from build123d import *

# Parameters (mm, degrees)
SKETCH1_W            = 114.4
SKETCH1_H            = 94.4
BOSS_EXTRUDE1_DEPTH  = 10
SHELL2_T             = -2
FILLET3_R            = 5
FILLET4_R            = 5
SKETCH5_R            = 4
BOSS_EXTRUDE12_DEPTH = 8
FILLET5_R            = 5
FILLET6_R            = 5
FILLET7_R            = 5
FILLET8_R            = 5
FILLET9_R            = 5
FILLET10_R           = 5
FILLET11_DEPTH       = 9
FILLET12_DEPTH       = 9
SKETCH6_R            = 1.6
CUT_EXTRUDE1_DEPTH   = 10
SKETCH7_R            = 4
BOSS_EXTRUDE13_DEPTH = 10
SKETCH8_R            = 1.5
CUT_EXTRUDE2_DEPTH   = 8
SKETCH9_R            = 2.5
CUT_EXTRUDE3_DEPTH   = 2


with BuildPart() as part:
    # Sketch1 → Boss-Extrude1 (new body)
    with BuildSketch(Plane(origin=(0, 0, 0), x_dir=(1, 0, 0), z_dir=(0, 1, 0))):
        with Locations((57.2, 47.2)):
            Rectangle(SKETCH1_W, SKETCH1_H)
    extrude(amount=BOSS_EXTRUDE1_DEPTH)

    # Shell2
    shell2_openings = [part.faces().sort_by_distance(p)[0] for p in [
        (57.2, 0, -47.2),
    ]]
    offset(amount=SHELL2_T, openings=shell2_openings, kind=Kind.INTERSECTION)

    # Fillet3
    fillet3_edges = [part.edges().sort_by_distance(p)[0] for p in [
        (0, 5, -94.4),
        (114.4, 5, -94.4),
        (114.4, 5, 0),
        (0, 5, 0),
    ]]
    fillet(fillet3_edges, radius=FILLET3_R)

    # Fillet4
    fillet4_edges = [part.edges().sort_by_distance(p)[0] for p in [
        (2, 4, -92.4),
        (2, 4, -2),
        (112.4, 4, -2),
        (112.4, 4, -92.4),
    ]]
    fillet(fillet4_edges, radius=FILLET4_R)

    # Sketch5 → Boss-Extrude12 (add)
    with BuildSketch(Plane(origin=(0, 8, 0), x_dir=(-1, 0, 0), z_dir=(0, -1, 0))):
        with Locations((-108.4, 6)):
            Circle(SKETCH5_R)
        with Locations((-108.4, 88.4)):
            Circle(SKETCH5_R)
        with Locations((-6, 88.4)):
            Circle(SKETCH5_R)
        with Locations((-6, 6)):
            Circle(SKETCH5_R)
    extrude(amount=BOSS_EXTRUDE12_DEPTH)

    # Fillet5
    # the kernel refuses this fillet: 5 mm, written as the material it adds along each edge
    with BuildSketch(Plane(origin=(112.372048604, 0, -6.472048604), x_dir=(-0.783459029597643, 0, -0.6214434398574978), z_dir=(0, 1, 0))) as fillet5_piece_1_section:
        with BuildLine():
            CenterArc((9.160403969, -3.547792862), FILLET5_R, 134.800989095, 83.620629792)
            Line((5.243108821, -6.655010061), (4.851379306, -6.965731781))
            ThreePointArc((4.851379306, -6.965731781), (-0.085536357, -0.74172022), (-0.422348831, -0.26762187))
            Line((-0.422348831, -0.26762187), (0.35232323, 0.354779286))
            ThreePointArc((0.35232323, 0.354779286), (2.818585837, -0.661765711), (5.284848444, 0.354779286))
            Line((5.284848444, 0.354779286), (5.637171673, 0))
        make_face()
    fillet5_piece_1 = extrude(amount=29.180673535, mode=Mode.PRIVATE)
    fillet5_piece_1 = split(fillet5_piece_1, bisect_by=Plane(origin=(112.372048604, 10, -6.472048604), z_dir=(0, -1, 0)), keep=Keep.TOP, mode=Mode.PRIVATE)
    add(fillet5_piece_1)

    # Fillet6
    # the kernel refuses this fillet: 5 mm, written as the material it adds along each edge
    with BuildSketch(Plane(origin=(107.927951396, 0, -2.027951396), x_dir=(-0.6214434398574917, 0, -0.7834590295976479), z_dir=(0, 1, 0))) as fillet6_piece_1_section:
        with BuildLine():
            CenterArc((9.160403969, 3.547792862), FILLET6_R, 141.578381114, 83.620629792)
            Line((5.243108821, 6.655010061), (4.851379306, 6.965731781))
            ThreePointArc((4.851379306, 6.965731781), (-0.085536357, 0.74172022), (-0.422348831, 0.26762187))
            Line((-0.422348831, 0.26762187), (0.35232323, -0.354779286))
            ThreePointArc((0.35232323, -0.354779286), (2.818585837, 0.661765711), (5.284848444, -0.354779286))
            Line((5.284848444, -0.354779286), (5.637171673, 0))
        make_face()
    fillet6_piece_1 = extrude(amount=29.180673535, mode=Mode.PRIVATE)
    fillet6_piece_1 = split(fillet6_piece_1, bisect_by=Plane(origin=(107.927951396, 10, -2.027951396), z_dir=(0, -1, 0)), keep=Keep.TOP, mode=Mode.PRIVATE)
    add(fillet6_piece_1)

    # Fillet7
    # the kernel refuses this fillet: 5 mm, written as the material it adds along each edge
    with BuildSketch(Plane(origin=(112.372048604, 0, -87.927951396), x_dir=(-0.783459029597643, 0, 0.6214434398574978), z_dir=(0, 1, 0))) as fillet7_piece_1_section:
        with BuildLine():
            CenterArc((9.160403969, 3.547792862), FILLET7_R, 141.578381114, 83.620629792)
            Line((5.243108821, 6.655010061), (4.851379306, 6.965731781))
            ThreePointArc((4.851379306, 6.965731781), (-0.085536357, 0.74172022), (-0.422348831, 0.26762187))
            Line((-0.422348831, 0.26762187), (0.35232323, -0.354779286))
            ThreePointArc((0.35232323, -0.354779286), (2.818585837, 0.661765711), (5.284848444, -0.354779286))
            Line((5.284848444, -0.354779286), (5.637171673, 0))
        make_face()
    fillet7_piece_1 = extrude(amount=29.180673535, mode=Mode.PRIVATE)
    fillet7_piece_1 = split(fillet7_piece_1, bisect_by=Plane(origin=(112.372048604, 10, -87.927951396), z_dir=(0, -1, 0)), keep=Keep.TOP, mode=Mode.PRIVATE)
    add(fillet7_piece_1)

    # Fillet8
    # the kernel refuses this fillet: 5 mm, written as the material it adds along each edge
    with BuildSketch(Plane(origin=(107.927951396, 0, -92.372048604), x_dir=(-0.6214434398574917, 0, 0.7834590295976479), z_dir=(0, 1, 0))) as fillet8_piece_1_section:
        with BuildLine():
            CenterArc((9.160403969, -3.547792862), FILLET8_R, 134.800989095, 83.620629792)
            Line((5.243108821, -6.655010061), (4.851379306, -6.965731781))
            ThreePointArc((4.851379306, -6.965731781), (-0.085536357, -0.74172022), (-0.422348831, -0.26762187))
            Line((-0.422348831, -0.26762187), (0.35232323, 0.354779286))
            ThreePointArc((0.35232323, 0.354779286), (2.818585837, -0.661765711), (5.284848444, 0.354779286))
            Line((5.284848444, 0.354779286), (5.637171673, 0))
        make_face()
    fillet8_piece_1 = extrude(amount=29.180673535, mode=Mode.PRIVATE)
    fillet8_piece_1 = split(fillet8_piece_1, bisect_by=Plane(origin=(107.927951396, 10, -92.372048604), z_dir=(0, -1, 0)), keep=Keep.TOP, mode=Mode.PRIVATE)
    add(fillet8_piece_1)

    # Fillet9
    # the kernel refuses this fillet: 5 mm, written as the material it adds along each edge
    with BuildSketch(Plane(origin=(6.472048604, 29.180673535, -2.027951396), x_dir=(0.9999945577477605, 0, 0.003299162751511756), z_dir=(0, -1, 0))) as fillet9_piece_1_section:
        with BuildLine():
            CenterArc((8.4557736, -4.999972789), FILLET9_R, 89.810971555, 83.620629792)
            Line((3.488593561, -4.428026585), (2.991875557, -4.370831965))
            ThreePointArc((2.991875557, -4.370831965), (2.264117061, -1.804476076), (-0.060643809, -0.496308703))
            Line((-0.060643809, -0.496308703), (-0.051154492, 0.497376334))
            ThreePointArc((-0.051154492, 0.497376334), (0.52969032, 0.526206725), (8.473918995, 0.499997279))
            Line((8.473918995, 0.499997279), (8.472269414, 0))
        make_face()
    fillet9_piece_1 = extrude(amount=29.180673535, mode=Mode.PRIVATE)
    fillet9_piece_1 = split(fillet9_piece_1, bisect_by=Plane(origin=(6.472048604, 10, -2.027951396), z_dir=(0, -1, 0)), keep=Keep.TOP, mode=Mode.PRIVATE)
    add(fillet9_piece_1)

    # Fillet10
    # the kernel refuses this fillet: 5 mm, written as the material it adds along each edge
    with BuildSketch(Plane(origin=(2.027951396, 29.180673535, -6.472048604), x_dir=(0.783459029597646, 0, -0.6214434398574942), z_dir=(0, -1, 0))) as fillet10_piece_1_section:
        with BuildLine():
            CenterArc((9.160403969, -3.547792862), FILLET10_R, 134.800989095, 83.620629792)
            Line((5.243108821, -6.655010061), (4.851379306, -6.965731781))
            ThreePointArc((4.851379306, -6.965731781), (-0.085536357, -0.74172022), (-0.422348831, -0.26762187))
            Line((-0.422348831, -0.26762187), (0.35232323, 0.354779286))
            ThreePointArc((0.35232323, 0.354779286), (2.818585837, -0.661765711), (5.284848444, 0.354779286))
            Line((5.284848444, 0.354779286), (5.637171673, 0))
        make_face()
    fillet10_piece_1 = extrude(amount=29.180673535, mode=Mode.PRIVATE)
    fillet10_piece_1 = split(fillet10_piece_1, bisect_by=Plane(origin=(2.027951396, 10, -6.472048604), z_dir=(0, -1, 0)), keep=Keep.TOP, mode=Mode.PRIVATE)
    add(fillet10_piece_1)

    # Fillet11: read off the stored shape, not the designer's step
    # Fillet11 outline → Fillet11 (add)
    with BuildSketch(Plane(origin=(0, 0, 0), x_dir=(1, 0, 0), z_dir=(0, 1, 0))):
        with BuildLine():
            ThreePointArc((2, 79.45572809), (3.273220038, 82.789061423), (6.444444444, 84.42476804))
            ThreePointArc((6.444444444, 84.42476804), (3.51422624, 85.266163882), (2.027951396, 87.927951396))
            ThreePointArc((2.027951396, 87.927951396), (2.006992739, 87.664345398), (2, 87.4))
            Line((2, 87.4), (2, 79.45572809))
        make_face()
    extrude(amount=FILLET11_DEPTH)

    # Fillet12: read off the stored shape, not the designer's step
    # Fillet12 outline → Fillet12 (add)
    with BuildSketch(Plane(origin=(0, 0, 0), x_dir=(1, 0, 0), z_dir=(0, 1, 0))):
        with BuildLine():
            ThreePointArc((9.97523196, 87.955555556), (11.610938577, 91.126779962), (14.94427191, 92.4))
            Line((14.94427191, 92.4), (7, 92.4))
            ThreePointArc((7, 92.4), (6.735654602, 92.393007261), (6.472048604, 92.372048604))
            ThreePointArc((6.472048604, 92.372048604), (9.133836118, 90.88577376), (9.97523196, 87.955555556))
        make_face()
    extrude(amount=FILLET12_DEPTH)

    # Sketch6 → Cut-Extrude1 (cut)
    with BuildSketch(Plane(origin=(0, 0, 0), x_dir=(-1, 0, 0), z_dir=(0, -1, 0))):
        with Locations(Location((-6, 6, 0), (0, 0, 90))):
            Circle(SKETCH6_R)
        with Locations(Location((-108.4, 88.4, 0), (0, 0, 90))):
            Circle(SKETCH6_R)
        with Locations(Location((-108.4, 6, 0), (0, 0, 90))):
            Circle(SKETCH6_R)
        with Locations(Location((-6, 88.4, 0), (0, 0, 90))):
            Circle(SKETCH6_R)
    extrude(amount=-CUT_EXTRUDE1_DEPTH, mode=Mode.SUBTRACT)

    # Sketch7 → Boss-Extrude13 (add)
    with BuildSketch(Plane(origin=(0, 8, 0), x_dir=(-1, 0, 0), z_dir=(0, -1, 0))):
        with Locations(Location((-96.5, 19.1, 0), (0, 0, 90))):
            Circle(SKETCH7_R)
        with Locations(Location((-17, 19.1, 0), (0, 0, 90))):
            Circle(SKETCH7_R)
        with Locations(Location((-96.5, 77.4, 0), (0, 0, 90))):
            Circle(SKETCH7_R)
        with Locations(Location((-17, 77.4, 0), (0, 0, 90))):
            Circle(SKETCH7_R)
    extrude(amount=BOSS_EXTRUDE13_DEPTH)

    # Sketch8 → Cut-Extrude2 (cut)
    with BuildSketch(Plane(origin=(0, -2, 0), x_dir=(-1, 0, 0), z_dir=(0, -1, 0))):
        with Locations(Location((-17, 19.1, 0), (0, 0, 90))):
            Circle(SKETCH8_R)
        with Locations(Location((-96.5, 19.1, 0), (0, 0, 90))):
            Circle(SKETCH8_R)
        with Locations(Location((-96.5, 77.4, 0), (0, 0, 90))):
            Circle(SKETCH8_R)
        with Locations(Location((-17, 77.4, 0), (0, 0, 90))):
            Circle(SKETCH8_R)
    extrude(amount=-CUT_EXTRUDE2_DEPTH, mode=Mode.SUBTRACT)

    # Sketch9 → Cut-Extrude3 (cut)
    with BuildSketch(Plane(origin=(0, 10, 0), x_dir=(1, 0, 0), z_dir=(0, 1, 0))):
        with Locations(Location((6, 88.4, 0), (0, 0, 270))):
            Circle(SKETCH9_R)
        with Locations(Location((6, 6, 0), (0, 0, 270))):
            Circle(SKETCH9_R)
        with Locations(Location((108.4, 6, 0), (0, 0, 270))):
            Circle(SKETCH9_R)
        with Locations(Location((108.4, 88.4, 0), (0, 0, 270))):
            Circle(SKETCH9_R)
    extrude(amount=-CUT_EXTRUDE3_DEPTH, mode=Mode.SUBTRACT)


solid = part.part
Geometry check sheet. Reference: the model listing, model coordinates, mm. A direction names the side the tool comes from. Round coordinates to 2 decimals unless told otherwise and drop trailing zeros. Write each loop counter-clockwise with the first axis right and the second up, starting at its lowest first coordinate (ties: lowest second). Pieces come first, ordered by that corner, then holes. Notation, with made-up numbers: (18, 48) -> (75, 48) arc R11 ccw to (75, 53) -> close; hole circle Ø7 at (30.5, -25). An arc over 180 degrees is marked (long way). One line per item, written item: value. Start each with the question number.
(1) Cross-section at B-B, the plane z = -25.5. Record the cut outline in (x, y).
(2) Access from +Z, -Z, +X, -X, +Y, -Y to the whole of each face (thin tool, end or side, straight path). Record for faces 1 (the flat face through (94.8, -2, -19)), 2 (the cylindrical face through (107.44, 9.01, -86.09)), 3 (the flat face through (2, 4, -47)).
(3) Go/stop test with flat-tipped pins: pin 1 Ø0.9 at (x, z) = (97, -19.5) entering from -Y; pin 2 Ø8 at (x, z) = (6, -88.4) entering from -Y; pin 3 Ø2.5 at (x, z) = (108.5, -89.5) entering from +Y. Record where each tip stops, or that it passes through.
(4) Cross-section at D-D, the plane x = 69. Record the cut outline in (y, z), and give its area (3 significant figures).
(5) Draft check along Z on faces 4 (the cylindrical face through (92.951, 3.07, -79.246)), 5 (the flat face through (15, -2, -19)), 6 (the flat face through (56, 5, -94.4)). Enter one of: +Z half, -Z half, draft (parallel to the pull), parting line (faces both ways), or undercut.
(6) Cross-section at C-C, the plane y = 2. Give the number of separate pieces and of enclosed holes in the cut face, and give its area (3 significant figures).
(7) Cross-section at A-A, the plane x = 96.5. Record the cut outline in (y, z), and give its area (3 significant figures).
(8) Scan lines: line 1 (X direction, y = 8.65, z = -88.4); line 2 (X direction, y = 0.25, z = -67); line 3 (X direction, y = 4, z = -88.4). Record each from-to range of solid material in increasing order. Write a range as [from, to].
Answer:
1. outline: (0, 0) -> (2, 0) -> (2, 8) -> (112.4, 8) -> (112.4, 0) -> (114.4, 0) -> (114.4, 10) -> (0, 10) -> close
2. face 1: +Z, -Z, +X, -X, -Y
2. face 2: +Y
2. face 3: -Y
3. pin 1: y = 6
3. pin 2: y = 0
3. pin 3: y = 8
4. outline: (0, -94.4) -> (10, -94.4) -> (10, 0) -> (0, 0) -> (0, -2) -> (8, -2) -> (8, -92.4) -> (0, -92.4) -> close
4. area: 221 mm²
5. face 4: undercut
5. face 5: draft
5. face 6: -Z half
6. separate pieces: 5
6. enclosed holes: 9
6. area: 1,220 mm²
7. outline: (-2, -81.4) -> (8, -81.4) -> (8, -92.4) -> (0, -92.4) -> (0, -94.4) -> (10, -94.4) -> (10, 0) -> (0, 0) -> (0, -2) -> (8, -2) -> (8, -15.1) -> (-2, -15.1) -> (-2, -17.6) -> (6, -17.6) -> (6, -20.6) -> (-2, -20.6) -> (-2, -23.1) -> (8, -23.1) -> (8, -73.4) -> (-2, -73.4) -> (-2, -75.9) -> (6, -75.9) -> (6, -78.9) -> (-2, -78.9) -> close
7. area: 333 mm²
8. line 1: [0, 3.5], [8.5, 105.9], [110.9, 114.4]
8. line 2: [0, 2], [112.4, 114.4]
8. line 3: [0, 4.4], [7.6, 10.05], [104.35, 106.8], [110, 114.4]
